from build123d import *

# Parameters (mm, degrees)
BOSS_EXTRU_1_DEPTH = 96.8
CHANFREIN1_SIZE    = 1
CHANFREIN2_SIZE    = 3


with BuildPart() as part:
    # Esquisse1 → Boss.-Extru.1 (new body)
    with BuildSketch(Plane.XY):
        Polygon((-11.2, 0), (11.2, 0), (14.2, 3), (-14.2, 3), align=None)
    extrude(amount=BOSS_EXTRU_1_DEPTH)

    # Chanfrein1
    chanfrein1_edges = [part.edges().sort_by_distance(p)[0] for p in [
        (-12.7, 1.5, 96.8),
        (0, 0, 96.8),
        (12.7, 1.5, 96.8),
        (0, 3, 96.8),
    ]]
    chamfer(chanfrein1_edges, length=CHANFREIN1_SIZE)

    # Chanfrein2
    chanfrein2_edges = [part.edges().sort_by_distance(p)[0] for p in [
        (0, 0, 0),
    ]]
    chamfer(chanfrein2_edges, length=CHANFREIN2_SIZE - 0.0001)  # a hair under: the kernel refuses the full size


solid = part.part
Here's how the part is built. I have some questions about the finished solid (model axes, mm). Give positions to 0.01 mm unless a question says otherwise; leave off trailing zeros. Write each loop counter-clockwise with the first axis right and the second up, starting at its lowest first coordinate (ties: lowest second). Pieces come first, ordered by that corner, then holes. Notation, with made-up numbers: (-5, 56) -> (37, 56) arc R26 ccw to (37, 77) -> close; hole circle Ø5 at (-4, 46.25). An arc over 180 degrees is marked (long way). Use one line per item in the form item = value. Start each with the question number.
1. Will this pin go through, and if not, where does the flat tip stop? pin 1 Ø1 at (y, z) = (1.5, 76) entering from +X.
2. Imagine slicing it at B-B on z = 46. List the corners of the cut face in (x, y) for me, plus the area to 3 significant figures.
3. If I drill on L1, parallel to Z at x = -3.75, y = 0.2; L2, parallel to X at y = 0.6, z = 6; L3, parallel to Z at x = 5, y = 0.3, over which ranges is the centre line in solid material (lowest first)?
Entries:
q1.pin_1 = 13.2
q2.outline = (-14.2, 3) -> (-11.2, 0) -> (11.2, 0) -> (14.2, 3) -> close
q2.area = 76.2 mm²
q3.L1 = 2.8 to 96
q3.L2 = -11.8 to 11.8
q3.L3 = 2.7 to 96.1
